Part model, mm, in its own coordinate system. Face numbers are marked on the shaded views. A direction names the side the tool comes from. Round coordinates to 2 decimals unless told otherwise and drop trailing zeros. Write each loop counter-clockwise with the first axis right and the second up, starting at its lowest first coordinate (ties: lowest second). Pieces come first, ordered by that corner, then holes. Notation, with made-up numbers: M -26.5,58.5 L -13.5,58.5 A31 cw -13.5,97.5 Z; hole C -35,24 d11. An arc over 180 degrees is marked long. Use one line per item in the form item = value. Start each with the question number.
Item 1: Flat gauge pins, fed straight in: pin 1 Ø0.8 at (x, y) = (64.5, 11) entering from +Z; pin 2 Ø2 at (x, y) = (38.5, 5.5) entering from +Z; pin 3 Ø2.5 at (x, y) = (64.5, 12) entering from +Z. Where does each tip first touch, or does it go through?
Item 2: Mould opens along Y. For the marked faces 3, 4, 5 and 6 say: +Y half, -Y half, draft (parallel to the pull), parting line (faces both ways), or undercut.
Item 3: Cut at C-C, the plane y = 0. Give the cut face in (x, z).
Item 4: Cut at B-B, the plane x = 56. Give the cut face in (y, z).
Item 5: Cut at D-D, the plane x = 48. Give the cut face in (y, z).
Item 6: Cut at A-A, the plane z = 4.25. State how many separate pieces and enclosed holes the cut face has, then the cut area to 3 significant figures.
Item 7: Probe L1, parallel to X at y = 8, z = 0.2; L2, parallel to X at y = 0, z = 0.25; L3, parallel to Y at x = 56, z = 0.2. List the from-to ranges inside material, lowest first.
Item 8: Which spindle directions (+Z, -Z, +X, -X, +Y, -Y) get a long thin tool onto all of the face, cutting with end or side? Do the marked faces 1 and 2. Say none if no direction does.
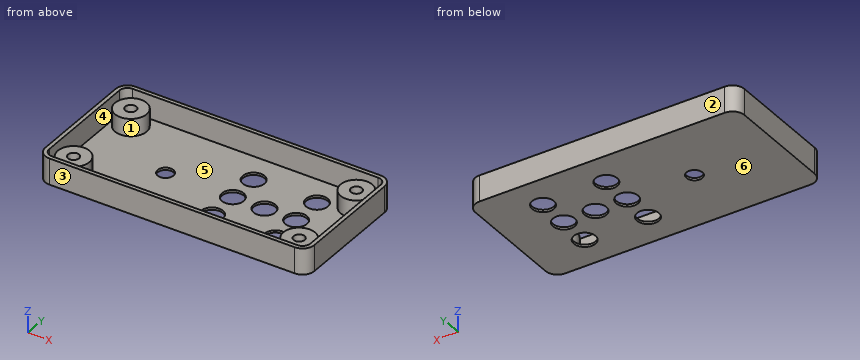
Autodesk Fusion 360 part; units mm, degrees
sketch "Skizze1" plane through (0, 0, 0) normal (0, 0, 1) x (1, 0, 0)
  line L0 (1.5, 0) -> (69.5, 0)
  line L1 (69.5, 0) -> (69.5, 16.5)
  line L2 (69.5, 16.5) -> (1.5, 16.5)
  line L3 (1.5, 16.5) -> (1.5, 0)
  dimension "d1" = 68
  dimension "d2" = 16.5
extrude "Extrusion1" add sketch "Skizze1" along normal blind 0.6
sketch "Skizze2" plane through (0, 0, 0.6) normal (0, 0, 1) x (-1, 0, 0)
  line L0 (-1.5, -16.5) -> (-1.5, 0)
  line L1 (-1.5, 0) -> (-69.5, 0)
  line L2 (-69.5, 0) -> (-69.5, -16.5)
  line L3 (-69.5, -16.5) -> (-1.5, -16.5)
  line L4 (-1.5, 0) -> (-1.5, -16.5)
  line L5 (-1.5, -16.5) -> (-69.5, -16.5)
  line L6 (-69.5, -16.5) -> (-69.5, 0)
  line L7 (-69.5, 0) -> (-68.5, 0)
  line L8 (-68.5, 0) -> (-68.5, -15.5)
  line L9 (-68.5, -15.5) -> (-2.5, -15.5)
  line L10 (-2.5, -15.5) -> (-2.5, 0)
  line L11 (-2.5, 0) -> (-1.5, 0)
  dimension "d5" = 1
  dimension "d6" = 1
  dimension "d7" = 1
extrude "Extrusion2" add sketch "Skizze2" along normal blind 6 contours L0 L1 L2 L3 L4 L5 L6 L7 L8 L9 L10 L11
fillet "Abrundung1" radius 2 2 edges at (2.5, 15.5, 3.6) (68.5, 15.5, 3.6)
fillet "Abrundung2" radius 3 2 edges at (69.5, 16.5, 3.3) (1.5, 16.5, 3.3)
sketch "Skizze3" plane through (0, 0, 0.6) normal (0, 0, 1) x (-1, 0, 0)
  arc A0 (-68.5, -13.5) -> (-66.5, -15.5) centre (-66.5, -13.5) ccw
  line L0 (-66.5, -15.5) -> (-4.5, -15.5)
  arc A1 (-4.5, -15.5) -> (-2.5, -13.5) centre (-4.5, -13.5) ccw
  line L1 (-2.5, -13.5) -> (-2.5, 0)
  line L2 (-2.5, 0) -> (-68.5, 0)
  line L3 (-68.5, 0) -> (-68.5, -13.5)
  circle A2 centre (-64, -11) radius 4
  circle A3 centre (-7, -11) radius 4
  dimension "d14" = 8
  dimension "d15" = 8
  dimension "d16" = 57
  dimension "d17" = 11
  dimension "d18" = 7
  dimension "d19" = 11
extrude "Extrusion3" add sketch "Skizze3" along normal blind 4.4 contours A2 | A3
sketch "Skizze4" plane through (0, 0, 5) normal (0, 0, 1) x (-1, 0, 0)
  circle A0 centre (-7, -11) radius 4
  circle A1 centre (-64, -11) radius 4
  point P0 (-7, -11)
  point P1 (-64, -11)
hole "Bohrung1" at (7, 11, 5) at (64, 11, 5) direction (0, 0, -1) diameter 2.8 depth 4 tip angle 180
sketch "Skizze5" plane through (0, 0, 0.6) normal (0, 0, 1) x (-1, 0, 0)
  circle A0 centre (-64, -11) radius 4
  circle A1 centre (-7, -11) radius 4
  arc A2 (-68.5, -13.5) -> (-66.5, -15.5) centre (-66.5, -13.5) ccw
  line L0 (-66.5, -15.5) -> (-4.5, -15.5)
  arc A3 (-4.5, -15.5) -> (-2.5, -13.5) centre (-4.5, -13.5) ccw
  line L1 (-2.5, -13.5) -> (-2.5, 0)
  line L2 (-2.5, 0) -> (-68.5, 0)
  line L3 (-68.5, 0) -> (-68.5, -13.5)
  circle A4 centre (-48, 0) radius 2.75
  circle A5 centre (-56, 0) radius 2.75
  circle A6 centre (-56, -8) radius 2.75
  circle A7 centre (-40, -8) radius 2.75
  circle A8 centre (-40, 0) radius 2.75
  circle A9 centre (-23, 0) radius 2
  dimension "d25" = 4
  dimension "d26" = 5.5
  dimension "d27" = 5.5
  dimension "d28" = 5.5
  dimension "d29" = 5.5
  dimension "d30" = 5.5
  dimension "d31" = 8
  dimension "d32" = 8
  dimension "d33" = 8
  dimension "d34" = 8
  dimension "d36" = 48
  dimension "d37" = 8
  dimension "d38" = 8
  dimension "d43" = 17
extrude "Extrusion4" cut sketch "Skizze5" against normal blind 5 contours L2 A5 | L2 A4 | L2 A9 | L2 A8 | A6 | A7 picked at (-55.1334, -0.6679) picked at (-47.1334, -0.6679) picked at (-23.6445, -0.2959) picked at (-39.1334, -0.6679)
mirror "Spiegeln1" about plane through (0, 0, 0) normal (0, 1, 0) of bodies 1 merged
equation "d20 = 6 mm - 1.6 mm"
Model answer:
q1.pin_1 = 1
q1.pin_2 = 0.6
q1.pin_3 = 5
q2.face_3 = -Y half
q2.face_4 = undercut
q2.face_5 = undercut
q2.face_6 = draft
q3.outline = M 1.5,0 L 21,0 L 21,0.6 L 2.5,0.6 L 2.5,6.6 L 1.5,6.6 Z; M 25,0 L 37.25,0 L 37.25,0.6 L 25,0.6 Z; M 42.75,0 L 45.25,0 L 45.25,0.6 L 42.75,0.6 Z; M 50.75,0 L 53.25,0 L 53.25,0.6 L 50.75,0.6 Z; M 58.75,0 L 69.5,0 L 69.5,6.6 L 68.5,6.6 L 68.5,0.6 L 58.75,0.6 Z
q4.outline = M -16.5,0 L -10.75,0 L -10.75,0.6 L -15.5,0.6 L -15.5,6.6 L -16.5,6.6 Z; M -5.25,0 L -2.75,0 L -2.75,0.6 L -5.25,0.6 Z; M 2.75,0 L 5.25,0 L 5.25,0.6 L 2.75,0.6 Z; M 10.75,0 L 16.5,0 L 16.5,6.6 L 15.5,6.6 L 15.5,0.6 L 10.75,0.6 Z
q5.outline = M -16.5,0 L -2.75,0 L -2.75,0.6 L -15.5,0.6 L -15.5,6.6 L -16.5,6.6 Z; M 2.75,0 L 16.5,0 L 16.5,6.6 L 15.5,6.6 L 15.5,0.6 L 2.75,0.6 Z
q6.separate_pieces = 5
q6.enclosed_holes = 5
q6.area = 370 mm²
q7.L1 = 1.5 to 37.25, 42.75 to 53.25, 58.75 to 69.5
q7.L2 = 1.5 to 21, 25 to 37.25, 42.75 to 45.25, 50.75 to 53.25, 58.75 to 69.5
q7.L3 = -16.5 to -10.75, -5.25 to -2.75, 2.75 to 5.25, 10.75 to 16.5
q8.face_1 = +Z
q8.face_2 = +Z, -Z, +X, -X, +Y
